Model file for the job. Use its own axes, mm. Round coordinates to 2 decimals unless told otherwise and drop trailing zeros. Loops run counter-clockwise (first coordinate to the right, second up) from the corner with the lowest first, then second, coordinate; pieces in that order, holes last. Notation, with made-up numbers: M 46,74 L 86,74 A34 cw 86,107 Z; hole C -14,4 d10. An arc over 180 degrees is marked long. Use a Markdown table: item, result. Add a question column.
Item 1: Saw through at A-A on x = -30. Write the cut outline in (y, z).
Item 2: Saw through at D-D on y = 17. Write the cut outline in (x, z).
Item 3: Saw through at C-C on y = 1.5. Write the cut outline in (x, z), then the cut area to 3 significant figures.
Item 4: Saw through at B-B on z = 50. Write the cut outline in (x, y).
Item 5: Wall check: L1, parallel to Y at x = 38, z = 72; L2, parallel to Z at x = 12.5, y = 15; L3, parallel to Z at x = 27.5, y = -35.5. Give the ranges that are in metal, low to high. Write a range as from..to.
Item 6: Pin check, flat tips, straight feed: P1, Ø17, axis at x = 14.34, y = 13.59, coming from the -Z side; P2, Ø7.5, axis at x = 14, y = 10, coming from the -Z side; P3, Ø4.5, axis at x = 4.5, z = 49, coming from the +Y side; P4, Ø5, axis at x = 41.5, y = 24.5, coming from the +Z side. Stop position of each tip, or through.
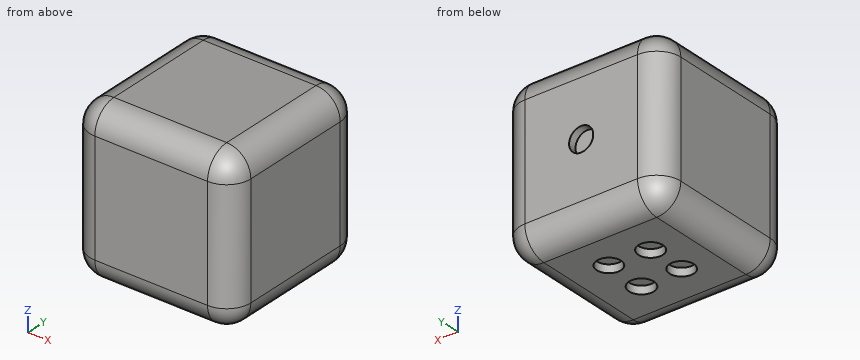
```python
from build123d import *

# Parameters (mm, degrees)
F0_W     = 100
F0_H     = 100
F1_DEPTH = 100
F2_R     = 15
F3_R     = 7.5
F4_DEPTH = 5
F5_R     = 7.5
F5_R_2   = 7.589466
F5_R_3   = 7.712973
F6_DEPTH = 5


with BuildPart() as f1:
    # F0 (on Top) → F1 (new body)
    with BuildSketch(Plane.XY):
        with Locations((2.459805, 0.276836)):
            Rectangle(F0_W, F0_H)
    extrude(amount=F1_DEPTH)

    # F2
    f2_edges = [f1.edges().sort_by_distance(p)[0] for p in [
        (2.459805, 50.276836, 0),
        (-47.540195, 50.276836, 50),
        (2.459805, 50.276836, 100),
        (52.459805, 50.276836, 50),
        (-47.540195, 0.276836, 0),
        (2.459805, -49.723164, 0),
        (52.459805, 0.276836, 0),
        (-47.540195, -49.723164, 50),
        (-47.540195, 0.276836, 100),
        (52.459805, 0.276836, 100),
        (52.459805, -49.723164, 50),
        (2.459805, -49.723164, 100),
    ]]
    fillet(f2_edges, radius=F2_R)

    # F3 (on face) → F4 (cut)
    with BuildSketch(Plane(origin=(0, 50.276836, 0), x_dir=(-1, 0, 0), z_dir=(0, 1, 0))):
        with Locations((-2.459805, 50)):
            Circle(F3_R)
    extrude(amount=-F4_DEPTH, mode=Mode.SUBTRACT)

    # F5 (on face) → F6 (cut)
    with BuildSketch(Plane(origin=(0, 0, 0), x_dir=(1, 0, 0), z_dir=(0, 0, -1))):
        with Locations((14.340434, -13.589303)):
            Circle(F5_R)
        with Locations((-10.799815, -12.571245)):
            Circle(F5_R_2)
        with Locations((14.473066, 12.134452)):
            Circle(F5_R_3)
        with Locations((-11.385111, 10.983491)):
            Circle(F5_R)
    extrude(amount=-F6_DEPTH, mode=Mode.SUBTRACT)


solid = f1.part
```
Entries:
| question | item | result |
|---|---|---|
| 1 | outline | M -49.72,15 A15 ccw -34.72,0 L 35.28,0 A15 ccw 50.28,15 L 50.28,85 A15 ccw 35.28,100 L -34.72,100 A15 ccw -49.72,85 Z |
| 2 | outline | M -47.54,15 A15 ccw -32.54,0 L -16.96,0 L -16.96,5 L -4.64,5 L -4.64,0 L 7.66,0 L 7.66,5 L 21.02,5 L 21.02,0 L 37.46,0 A15 ccw 52.46,15 L 52.46,85 A15 ccw 37.46,100 L -32.54,100 A15 ccw -47.54,85 Z |
| 3 | outline | M -47.54,15 A15 ccw -32.54,0 L 37.46,0 A15 ccw 52.46,15 L 52.46,85 A15 ccw 37.46,100 L -32.54,100 A15 ccw -47.54,85 Z |
| 3 | area | 9,810 mm2 |
| 4 | outline | M -47.54,-34.72 A15 ccw -32.54,-49.72 L 37.46,-49.72 A15 ccw 52.46,-34.72 L 52.46,35.28 A15 ccw 37.46,50.28 L 9.96,50.28 L 9.96,45.28 L -5.04,45.28 L -5.04,50.28 L -32.54,50.28 A15 ccw -47.54,35.28 Z |
| 5 | L1 | -49.71..50.27 |
| 5 | L2 | 5..100 |
| 5 | L3 | 0.02..99.98 |
| 6 | P1 | z = 0 |
| 6 | P2 | z = 5 |
| 6 | P3 | y = 45.28 |
| 6 | P4 | z = 99.92 |
